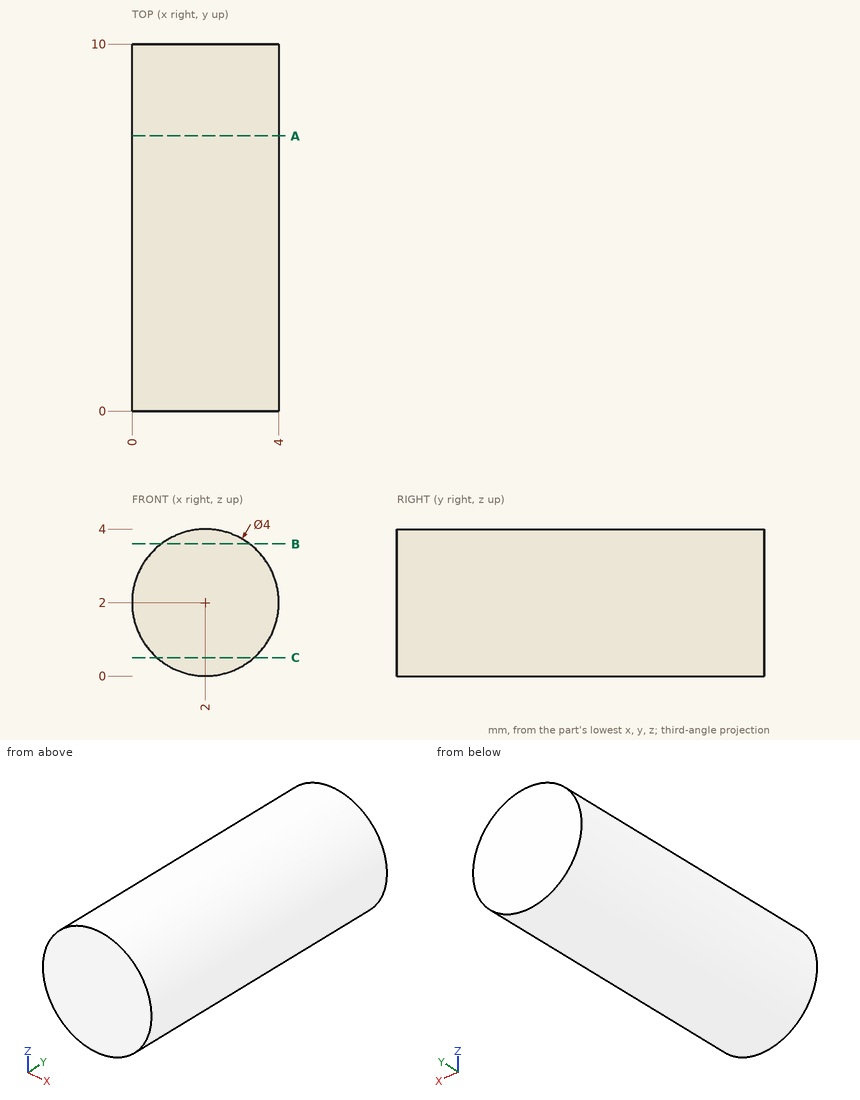
Part print with two shaded views. Sizes in mm from the minimum x, y, z corner. Round coordinates to 2 decimals unless told otherwise and drop trailing zeros. Loops run counter-clockwise (first coordinate to the right, second up) from the corner with the lowest first, then second, coordinate; pieces in that order, holes last. Notation, with made-up numbers: (-1.75, 28) - (16.25, 28) arc R13 cw to (16.25, 33) - close; hole circle Ø1 at (-25.75, -30). An arc over 180 degrees is marked (long way). Put each result on its own line as item: value.
1. Wall check: line 1 (Z direction, x = 0.9, y = 0.5); line 2 (X direction, y = 3.5, z = 1.4); line 3 (X direction, y = 1.25, z = 3.4). Give the ranges that are in metal, low to high.
Geometry check:
line 1: 0.33 to 3.67
line 2: 0.09 to 3.91
line 3: 0.57 to 3.43
2. Slice it at A-A on y = 7.5. List the corners of the cut face in (x, z).
Geometry check:
outline: circle Ø4 at (2, 2)
3. Slice it at C-C on z = 0.5. List the corners of the cut face in (x, y), and give its area (3 significant figures).
Geometry check:
outline: (0.68, 0) - (3.32, 0) - (3.32, 10) - (0.68, 10) - close
area: 26.5 mm²
4. Slice it at B-B on z = 3.6. List the corners of the cut face in (x, y).
Geometry check:
outline: (0.8, 0) - (3.2, 0) - (3.2, 10) - (0.8, 10) - close
